Verification items for this drawing (mm, ordinates from the low corner). A direction names the side the tool comes from. Give positions to 0.01 mm unless a question says otherwise; leave off trailing zeros. Loops run counter-clockwise (first coordinate to the right, second up) from the corner with the lowest first, then second, coordinate; pieces in that order, holes last. Notation, with made-up numbers: M 29.25,68 L 35.25,68 A31 ccw 35.25,102 Z; hole C -24.5,77 d6. An arc over 180 degrees is marked long. Put each result on its own line as item: value. Start each with the question number.
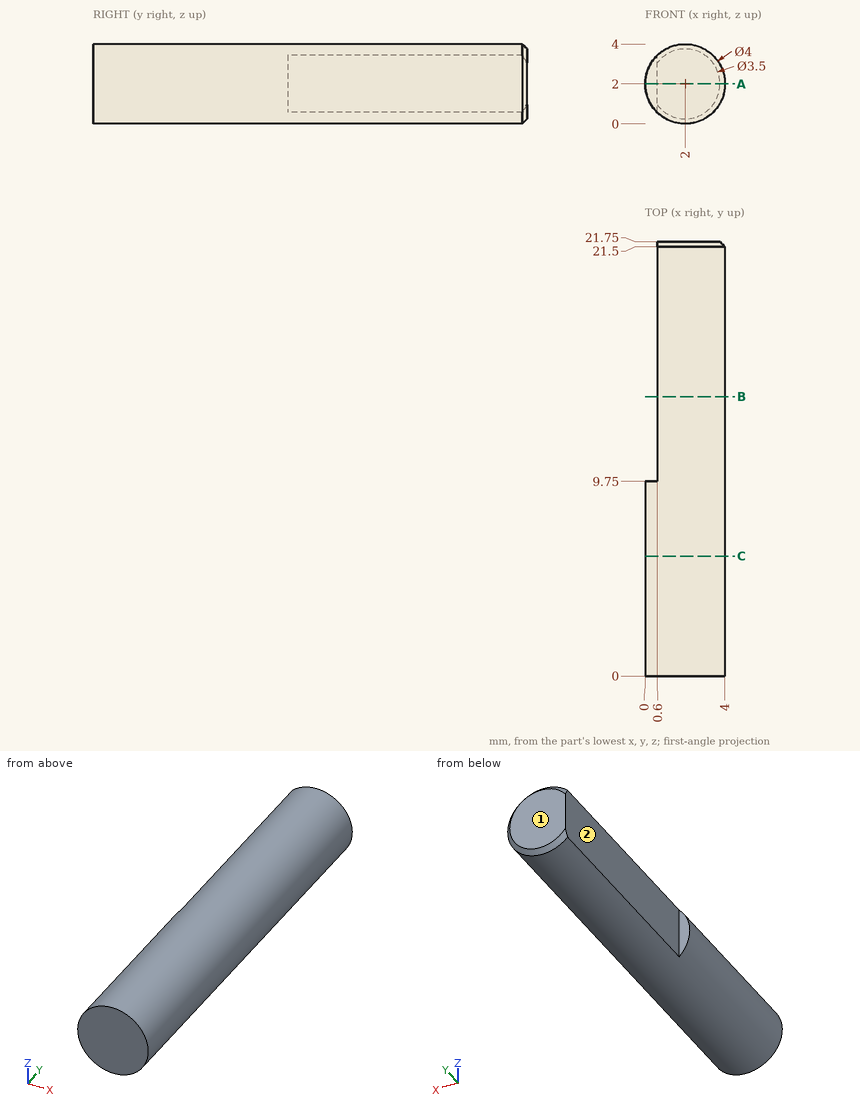
Q1. Scan lines: L1, parallel to Y at x = 0.2, z = 1.35; L2, parallel to Z at x = 1.25, y = 20; L3, parallel to Z at x = 1.6, y = 12.5. Record each from-to range of solid material in increasing order.
Q2. Cross-section at C-C, the plane y = 6. Record the boundary of the cut face in (x, z).
Q3. Go/stop test with a flat-tipped pin: pin 1 (1 mm diameter, centred on y = 10.5, z = 0.5, fed in from -X). Record where the tip stops, or that it passes through.
Q4. Set-up check for the marked faces 1 and 2: record each of +Z, -Z, +X, -X, +Y, -Y from which the full face is reachable in a straight line by a thin tool's end or side.
Q5. Cross-section at A-A, the plane z = 2. Record the boundary of the cut face in (x, y).
Q6. Cross-section at B-B, the plane y = 14. Record the boundary of the cut face in (x, z), then the cut area to 3 significant figures.
Ans:
1. L1: y = 0 to 9.75
1. L2: z = 0.15 to 3.85
1. L3: z = 0.04 to 3.96
2. outline: C 2,2 d4
3. pin 1: stops at x = 0.6
4. face 1: +Z, -Z, +X, -X, +Y
4. face 2: +Z, -Z, -X, +Y
5. outline: M 0,0 L 4,0 L 4,21.5 L 3.75,21.75 L 0.6,21.75 L 0.6,9.75 L 0,9.75 Z
6. outline: M 0.6,0.57 A2 ccw long 0.6,3.43 Z
6. area: 11.4 mm^2
